Verification items for the finished model (mm, model axes). A direction names the side the tool comes from. Coordinates: 2 decimals unless noted, no trailing zeros. Loops run counter-clockwise (first coordinate to the right, second up) from the corner with the lowest first, then second, coordinate; pieces in that order, holes last. Notation, with made-up numbers: (-39.75, 81) -> (6.25, 81) arc R30 cw to (6.25, 103) -> close; hole circle Ø10 at (21, 19.25). An arc over 180 degrees is marked (long way). Answer as a JSON object with one key per item and string values. Group by question number.
Q1. Cross-section at A-A on z = -4. Record the boundary of the cut face in (x, y), and give its area (3 significant figures).
Q2. Cross-section at B-B on y = 0.7. Give the number of separate pieces and of enclosed holes in the cut face, and give its area (3 significant figures).
Q3. Release check for a two-part mould opening along Z. For faces 4 (the flat face through (0, 0, 0)), 5 (the flat face through (0, 1, -18.2)), 6 (the cylindrical face through (-17.6, 0.8, -13.6)) record: released by +Z, released by -Z, zero draft, split by the parting line, or undercut.
Q4. Scan lines: L1, parallel to X at y = 0.4, z = -15.25 (3 decimals); L2, parallel to X at y = 0.4, z = 3.5; L3, parallel to X at y = 0.65, z = 12. Record each from-to range of solid material in increasing order.
Q5. Gauge pin test, flat end, axial feed: pin 1 Ø0.8 at (y, z) = (0.5, 3.5) entering from -X. Record the tip position at first contact, or that the pin passes through.
Q6. Set-up check for faces 1 (the flat face through (-13.7, 1, 0)), 2 (the flat face through (13.7, 1, 0)), 3 (the cylindrical face through (-17.14, 0.81, -17.3)): record each of +Z, -Z, +X, -X, +Y, -Y from which the full face is reachable in a straight line by a thin tool's end or side.
```python
from build123d import *

# Parameters (mm, degrees)
SKETCH1_R           = 1.625
BOSS_EXTRUDE1_DEPTH = 1.6
FILLET1_R           = 3
FILLET2_R           = 5


with BuildPart() as part:
    # Sketch1 → Boss-Extrude1 (new body)
    with BuildSketch(Plane(origin=(0, 0, 0), x_dir=(1, 0, 0), z_dir=(0, 1, 0))):
        Polygon((-18, 18.2), (-18, 12.1), (-13.7, 12.1), (-13.7, -12.1), (-18, -12.1), (-18, -18.2), (18, -18.2), (18, -12.1), (13.7, -12.1), (13.7, 12.1), (18, 12.1), (18, 18.2), align=None)
        with Locations(Location((15.25, -15.25, 0), (0, 0, 270))):
            Circle(SKETCH1_R, mode=Mode.SUBTRACT)
        with Locations(Location((15.25, 15.25, 0), (0, 0, 270))):
            Circle(SKETCH1_R, mode=Mode.SUBTRACT)
        with Locations(Location((-15.25, 15.25, 0), (0, 0, 270))):
            Circle(SKETCH1_R, mode=Mode.SUBTRACT)
        with Locations(Location((-15.25, -15.25, 0), (0, 0, 270))):
            Circle(SKETCH1_R, mode=Mode.SUBTRACT)
    extrude(amount=BOSS_EXTRUDE1_DEPTH)

    # Fillet1
    fillet1_edges = [part.edges().sort_by_distance(p)[0] for p in [
        (-18, 0.8, 18.2),
        (-18, 0.8, 12.1),
        (-18, 0.8, -12.1),
        (-18, 0.8, -18.2),
        (18, 0.8, -18.2),
        (18, 0.8, -12.1),
        (18, 0.8, 12.1),
        (18, 0.8, 18.2),
    ]]
    fillet(fillet1_edges, radius=FILLET1_R)

    # Fillet2
    fillet2_edges = [part.edges().sort_by_distance(p)[0] for p in [
        (13.7, 0.8, -12.1),
        (13.7, 0.8, 12.1),
        (-13.7, 0.8, 12.1),
        (-13.7, 0.8, -12.1),
    ]]
    fillet(fillet2_edges, radius=FILLET2_R)


solid = part.part
```
Computed values:
{
 "1": {"outline": "(-13.7, 0) -> (13.7, 0) -> (13.7, 1.6) -> (-13.7, 1.6) -> close", "area": "43.8 mm²"},
 "2": {"separate pieces": "1", "enclosed holes": "4", "area": "1,060 mm²"},
 "3": {"face 4": "zero draft", "face 5": "released by -Z", "face 6": "undercut"},
 "4": {"L1": "x = -18 to -16.875, -13.625 to 13.625, 16.875 to 18", "L2": "x = -13.7 to 13.7", "L3": "x = -15.69 to 15.69"},
 "5": {"pin 1": "stops at x = -13.7"},
 "6": {"face 1": "-X, +Y, -Y", "face 2": "+X, +Y, -Y", "face 3": "-Z, -X, +Y, -Y"}
}
